```python
from build123d import *

# Parameters (mm, degrees)
ESQUISSE1_R             = 5
ESQUISSE1_W             = 15
ESQUISSE1_H             = 30
ESQUISSE1_H_2           = 50
BOSS_EXTRU_1_DEPTH      = 15
ESQUISSE2_R             = 5
ESQUISSE2_W             = 34.887872932
ESQUISSE2_H             = 15
ESQUISSE2_W_2           = 15
ESQUISSE2_W_3           = 10
ENL_V_MAT_EXTRU_1_DEPTH = 358.421320013


with BuildPart() as part:
    # Esquisse1 → Boss.-Extru.1 (new body)
    with BuildSketch(Plane.XY):
        with BuildLine():
            Line((-200, -155), (200, -155))
            ThreePointArc((200, -155), (235.355339059, -140.355339059), (250, -105))
            Line((250, -105), (250, 105))
            ThreePointArc((250, 105), (235.355339059, 140.355339059), (200, 155))
            Line((200, 155), (100, 155))
            ThreePointArc((100, 155), (82.32233047, 162.32233047), (75, 180))
            Line((75, 180), (75, 230))
            ThreePointArc((75, 230), (67.67766953, 247.67766953), (50, 255))
            Line((50, 255), (-50, 255))
            ThreePointArc((-50, 255), (-67.67766953, 247.67766953), (-75, 230))
            Line((-75, 230), (-75, 180))
            ThreePointArc((-75, 180), (-82.32233047, 162.32233047), (-100, 155))
            Line((-100, 155), (-200, 155))
            ThreePointArc((-200, 155), (-235.355339059, 140.355339059), (-250, 105))
            Line((-250, 105), (-250, -105))
            ThreePointArc((-250, -105), (-235.355339059, -140.355339059), (-200, -155))
        make_face()
        with Locations((200, 120)):
            Circle(ESQUISSE1_R, mode=Mode.SUBTRACT)
        with Locations(Location((200, -120, 0), (0, 0, 180))):
            Circle(ESQUISSE1_R, mode=Mode.SUBTRACT)
        with Locations((-200, -120)):
            Circle(ESQUISSE1_R, mode=Mode.SUBTRACT)
        with Locations(Location((-200, 120, 0), (0, 0, 180))):
            Circle(ESQUISSE1_R, mode=Mode.SUBTRACT)
        with Locations((200, 0)):
            Rectangle(ESQUISSE1_W, ESQUISSE1_H, mode=Mode.SUBTRACT)
        with Locations((200, 70)):
            Rectangle(ESQUISSE1_W, ESQUISSE1_H_2, mode=Mode.SUBTRACT)
        with Locations((200, -70)):
            Rectangle(ESQUISSE1_W, ESQUISSE1_H_2, mode=Mode.SUBTRACT)
        with Locations((-200, -70)):
            Rectangle(ESQUISSE1_W, ESQUISSE1_H_2, mode=Mode.SUBTRACT)
        with Locations((-200, 0)):
            Rectangle(ESQUISSE1_W, ESQUISSE1_H, mode=Mode.SUBTRACT)
        with Locations((-200, 70)):
            Rectangle(ESQUISSE1_W, ESQUISSE1_H_2, mode=Mode.SUBTRACT)
        with BuildLine():
            Line((50, -17.321312087), (-50, -17.321312087))
            ThreePointArc((-50, -17.321312087), (-67.321312087, 0), (-50, 17.321312087))
            Line((-50, 17.321312087), (50, 17.321312087))
            ThreePointArc((50, 17.321312087), (67.321312087, 0), (50, -17.321312087))
        make_face(mode=Mode.SUBTRACT)
    extrude(amount=BOSS_EXTRU_1_DEPTH)

    # Esquisse2 → Enlèv. mat.-Extru.1 (cut, through all)
    with BuildSketch(Plane.XY.offset(15)):
        with Locations((50, 205)):
            Circle(ESQUISSE2_R)
        with Locations(Location((-50, 205, 0), (0, 0, 180))):
            Circle(ESQUISSE2_R)
        with Locations((77.443936466, 205)):
            Rectangle(ESQUISSE2_W, ESQUISSE2_H)
        with Locations((0, 247.5)):
            Rectangle(ESQUISSE2_W_2, ESQUISSE2_H)
        with Locations((-77.443936466, 205)):
            Rectangle(ESQUISSE2_W, ESQUISSE2_H)
        with Locations((0, 162.5)):
            Rectangle(ESQUISSE2_W_2, ESQUISSE2_H)
        with Locations((12.5, 222.5)):
            Rectangle(ESQUISSE2_W_3, ESQUISSE2_H)
        with Locations((-12.5, 222.5)):
            Rectangle(ESQUISSE2_W_3, ESQUISSE2_H)
        with Locations((12.5, 187.5)):
            Rectangle(ESQUISSE2_W_3, ESQUISSE2_H)
        with Locations((-12.5, 187.5)):
            Rectangle(ESQUISSE2_W_3, ESQUISSE2_H)
    extrude(amount=-ENL_V_MAT_EXTRU_1_DEPTH, mode=Mode.SUBTRACT)


solid = part.part
```
Geometry: final body of the model. Coordinates: model frame, mm. A direction names the side the tool comes from. Coordinates: 2 decimals unless noted, no trailing zeros. Loops run counter-clockwise (first coordinate to the right, second up) from the corner with the lowest first, then second, coordinate; pieces in that order, holes last. Notation, with made-up numbers: (-10, 0.5) -> (-2, 0.5) arc R18 ccw to (-2, 14.5) -> close; hole circle Ø4 at (-14.75, 89.5). An arc over 180 degrees is marked (long way). Use a Markdown table: item, result. Add a question column.
(1) Line query: line 1 along Y through (x, z) = (200, 8.5); line 2 along X through (y, z) = (221, 0.5); line 3 along Y through (x, z) = (50, 7.5). Output: solid intervals per line, ascending.
(2) Section query A-A, the plane y = -57. Return loops of the section in (x, z).
(3) Section query D-D, the plane x = 219. Return loops of the section in (y, z), plus the area to 3 significant figures.
(4) Mould query, pull axis X, two halves, no side actions, for faces 1 (the flat face through (75, 189, 7)), 2 (the flat face through (-149, 155, 7)), 3 (the flat face through (-200, -15, 7)). Classes: pulls with the +X half, pulls with the -X half, needs draft (parallel to the pull), parting line crosses it, or undercut.
(5) Pin query (flat end, axial travel): pin 1 Ø3 at (x, z) = (-142.5, 1.5) entering from +Y; pin 2 Ø7.5 at (y, z) = (225, 7) entering from -X; pin 3 Ø9 at (x, y) = (-200, -120) entering from +Z; pin 4 Ø7.5 at (x, z) = (-2.5, 4.5) entering from +Y. Return the tip coordinate at first contact, or that it passes through.
(6) Access query for faces 4 (the cylindrical face through (67.317, 0.381, 7.395)), 5 (the flat face through (67, 212.5, 8)), 6 (the cylindrical face through (234.964, -140.742, 7.395)), 7 (the flat face through (-60, 205, 8)). Directions: +Z, -Z, +X, -X, +Y, -Y. A direction counts if a zero-diameter tool reaches every point of the face in a straight line with its end or side. Return the directions, or none.
(7) Section query C-C, the plane x = 133.5. Return loops of the section in (y, z).
(8) Section query B-B, the plane z = 3. State how many separate pieces and enclosed holes the cut face has, plus the area to 3 significant figures.
Answer:
| question | item | result |
|---|---|---|
| 1 | line 1 | y = -155 to -125, -115 to -95, -45 to -15, 15 to 45, 95 to 115, 125 to 155 |
| 1 | line 2 | x = -75 to -17.5, -7.5 to 7.5, 17.5 to 75 |
| 1 | line 3 | y = -155 to -17.32, 17.32 to 200, 210 to 255 |
| 2 | outline | (-250, 0) -> (-207.5, 0) -> (-207.5, 15) -> (-250, 15) -> close; (-192.5, 0) -> (192.5, 0) -> (192.5, 15) -> (-192.5, 15) -> close; (207.5, 0) -> (250, 0) -> (250, 15) -> (207.5, 15) -> close |
| 3 | outline | (-151.25, 0) -> (151.25, 0) -> (151.25, 15) -> (-151.25, 15) -> close |
| 3 | area | 4,540 mm^2 |
| 4 | face 1 | pulls with the +X half |
| 4 | face 2 | needs draft |
| 4 | face 3 | undercut |
| 5 | pin 1 | stops at y = 155 |
| 5 | pin 2 | stops at x = -75 |
| 5 | pin 3 | passes through |
| 5 | pin 4 | stops at y = 240 |
| 6 | face 4 | +Z, -Z |
| 6 | face 5 | +Z, -Z, +X |
| 6 | face 6 | +Z, -Z, +X, -Y |
| 6 | face 7 | +Z, -Z, -X |
| 7 | outline | (-155, 0) -> (155, 0) -> (155, 15) -> (-155, 15) -> close |
| 8 | separate pieces | 1 |
| 8 | enclosed holes | 18 |
| 8 | area | 158,000 mm^2 |
